Part model, mm, in its own coordinate system. Face numbers are marked on the shaded views. A direction names the side the tool comes from. Coordinates: 2 decimals unless noted, no trailing zeros. Write each loop counter-clockwise with the first axis right and the second up, starting at its lowest first coordinate (ties: lowest second). Pieces come first, ordered by that corner, then holes. Notation, with made-up numbers: (-4.75, 24) -> (17.25, 24) arc R9 cw to (17.25, 38) -> close; hole circle Ø11 at (30.5, 85). An arc over 180 degrees is marked (long way). One line per question, with ' | ' between items. Start each with the question number.
Item 1: Two-plate mould, pull along Z, no slides. Class the marked faces 3, 4 and 5: pulls with the +Z half, pulls with the -Z half, needs draft (parallel to the pull), parting line crosses it, or undercut.
Item 2: 3-axis set-ups, long thin cutter, end or side, ignore diameter. For the marked faces 1 and 2: which of +Z, -Z, +X, -X, +Y, -Y reach the whole face in a straight line?
Item 3: Probe probe 1 along X at (y, z) = (4.5, 1); probe 2 along X at (y, z) = (7.65, 0.15); probe 3 along Y at (x, z) = (0.15, -1.25). List the from-to ranges inside material, lowest first. Write a range as [from, to].
Item 4: Saw through at C-C (y = 1.5). List the corners of the cut face in (x, z).
Item 5: Pin check, flat tips, straight feed: pin 1 (2 mm diameter, centred on x = 0.5, y = 5, fed in from +Z); pin 2 (1.5 mm diameter, centred on x = 0, z = 0.5, fed in from +Y). Stop position of each tip, or through.
Item 6: Saw through at D-D (z = 1.25). List the corners of the cut face in (x, y), and give its area (3 significant figures).
Item 7: Saw through at B-B (z = 2.25). List the corners of the cut face in (x, y).
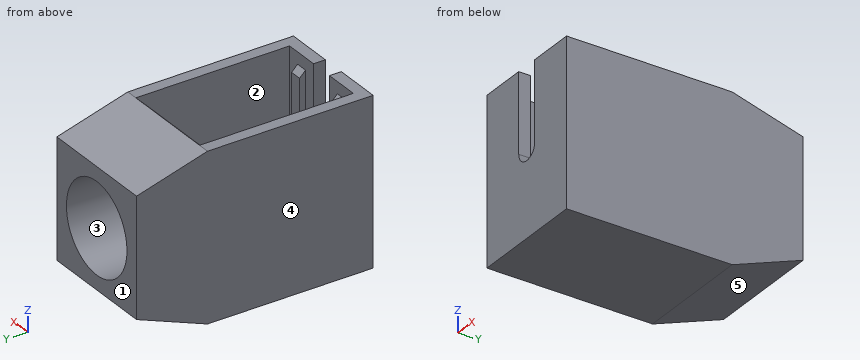
from build123d import *

# Parameters (mm, degrees)
SKETCH1_W           = 5
SKETCH1_H           = 7
BOSS_EXTRUDE1_DEPTH = 10
CUT_EXTRUDE1_DEPTH  = 12.715374514
SKETCH3_W           = 4
SKETCH3_H           = 6
CUT_EXTRUDE2_DEPTH  = 6.5
CUT_EXTRUDE3_REACH  = 12.886
SKETCH4_R           = 1.9
CUT_EXTRUDE4_REACH  = 12.886
SKETCH6_W           = 0.5
SKETCH6_H           = 6
BOSS_EXTRUDE3_DEPTH = 0.25
CHAMFER1_SIZE       = 0.25
CHAMFER2_SIZE       = 0.5


with BuildPart() as part:
    # Sketch1 → Boss-Extrude1 (new body)
    with BuildSketch(Plane(origin=(0, 0, 0), x_dir=(1, 0, 0), z_dir=(0, 1, 0))):
        Rectangle(SKETCH1_W, SKETCH1_H)
    extrude(amount=BOSS_EXTRUDE1_DEPTH)

    # Sketch2 → Cut-Extrude1 (cut, through all)
    with BuildSketch(Plane(origin=(2.5, 0, 0), x_dir=(0, 0, -1), z_dir=(1, 0, 0))):
        Polygon((-3.5, 7), (-2.65, 10), (-3.5, 10), align=None)
        Polygon((2.35, 10), (3.5, 10), (3.5, 7), align=None)
    extrude(amount=-CUT_EXTRUDE1_DEPTH, mode=Mode.SUBTRACT)

    # Sketch3 → Cut-Extrude2 (cut)
    with BuildSketch(Plane.XY.offset(3.5)):
        with Locations((0, 3.5)):
            Rectangle(SKETCH3_W, SKETCH3_H)
    extrude(amount=-CUT_EXTRUDE2_DEPTH, mode=Mode.SUBTRACT)

    # Sketch4 → Cut-Extrude3 (cut, up to next)
    with BuildSketch(Plane(origin=(0, 10, 0), x_dir=(1, 0, 0), z_dir=(0, 1, 0)), mode=Mode.PRIVATE) as cut_extrude3_sk1:
        with Locations(Location((0, -0.15, 0), (0, 0, 270))):
            Circle(SKETCH4_R)
    cut_extrude3_tool1 = extrude(cut_extrude3_sk1.sketch, amount=-CUT_EXTRUDE3_REACH, mode=Mode.PRIVATE) & part.part
    add(cut_extrude3_tool1.solids().sort_by_distance((0, 10, 0.15))[0], mode=Mode.SUBTRACT)

    # Sketch5 → Cut-Extrude4 (cut, up to next)
    with BuildSketch(Plane.XZ, mode=Mode.PRIVATE) as cut_extrude4_sk1:
        with BuildLine():
            Line((-0.5, 3.5), (-0.5, 0.15))
            ThreePointArc((-0.5, 0.15), (0, -0.35), (0.5, 0.15))
            Line((0.5, 0.15), (0.5, 3.5))
            Line((0.5, 3.5), (-0.5, 3.5))
        make_face()
    cut_extrude4_tool1 = extrude(cut_extrude4_sk1.sketch, amount=-CUT_EXTRUDE4_REACH, mode=Mode.PRIVATE) & part.part
    add(cut_extrude4_tool1.solids().sort_by_distance((0, 0, 1.626987))[0], mode=Mode.SUBTRACT)

    # Sketch6 → Boss-Extrude3 (add)
    with BuildSketch(Plane(origin=(0, 0.5, 0), x_dir=(1, 0, 0), z_dir=(0, 1, 0))):
        with Locations((-1.25, 0)):
            Rectangle(SKETCH6_W, SKETCH6_H)
        Polygon((1.5, 3), (1, 3), (1, -3), (1.5, -3), (1.5, 0), align=None)
    extrude(amount=BOSS_EXTRUDE3_DEPTH)

    # Chamfer1
    chamfer1_edges = [part.edges().sort_by_distance(p)[0] for p in [
        (1.25, 0.75, 3),
        (-1.25, 0.75, 3),
    ]]
    chamfer(chamfer1_edges, length=CHAMFER1_SIZE - 0.0001)  # a hair under: the kernel refuses the full size

    # Chamfer2
    chamfer2_edges = [part.edges().sort_by_distance(p)[0] for p in [
        (0, 6.5, 3.5),
    ]]
    chamfer(chamfer2_edges, length=CHAMFER2_SIZE - 0.0001)  # a hair under: the kernel refuses the full size


solid = part.part
From the geometry:
1) face 3: undercut | face 4: needs draft | face 5: pulls with the -Z half
2) face 1: +Z, -Z, +X, -X, +Y | face 2: +Z
3) probe 1: [-2.5, -2], [2, 2.5] | probe 2: [-2.5, -1.9], [1.9, 2.5] | probe 3: [0, 0.5]
4) outline: (-2.5, -3.5) -> (2.5, -3.5) -> (2.5, 3.5) -> (2, 3.5) -> (2, -3) -> (-2, -3) -> (-2, 3.5) -> (-2.5, 3.5) -> close
5) pin 1: z = -3 | pin 2: y = 0.5
6) outline: (-2.5, 0) -> (-0.5, 0) -> (-0.5, 0.5) -> (-1, 0.5) -> (-1, 0.75) -> (-1.5, 0.75) -> (-1.5, 0.5) -> (-2, 0.5) -> (-2, 6.5) -> (-1.55, 6.5) -> (-1.55, 10) -> (-2.5, 10) -> close; (0.5, 0) -> (2.5, 0) -> (2.5, 10) -> (1.55, 10) -> (1.55, 6.5) -> (2, 6.5) -> (2, 0.5) -> (1.5, 0.5) -> (1.5, 0.75) -> (1, 0.75) -> (1, 0.5) -> (0.5, 0.5) -> close | area: 14.9 mm2
7) outline: (-2.5, 0) -> (-0.5, 0) -> (-0.5, 0.5) -> (-1, 0.5) -> (-1, 0.75) -> (-1.5, 0.75) -> (-1.5, 0.5) -> (-2, 0.5) -> (-2, 6.5) -> (2, 6.5) -> (2, 0.5) -> (1.5, 0.5) -> (1.5, 0.75) -> (1, 0.75) -> (1, 0.5) -> (0.5, 0.5) -> (0.5, 0) -> (2.5, 0) -> (2.5, 10) -> (-2.5, 10) -> close
